from build123d import *

# Parameters (mm, degrees)
SKETCH_1_W          = 56
SKETCH_1_H          = 40
EXTRUDE_1_DEPTH     = 4
SKETCH_2_R          = 1.5
SKETCH_2_R_2        = 2.025
SKETCH_2_R_3        = 1.025
CUT_EXTRUDE_1_DEPTH = 34
EXTRUDE_2_DEPTH     = 4
SKETCH_4_R          = 1.525
CUT_EXTRUDE_2_DEPTH = 10
FILLET_1_R          = 2
CUT_EXTRUDE_3_DEPTH = 22
FILLET_2_R          = 2


with BuildPart() as part:
    # 草图1 → 凸台-拉伸1 (new body)
    with BuildSketch(Plane.XY):
        Rectangle(SKETCH_1_W, SKETCH_1_H)
    extrude(amount=EXTRUDE_1_DEPTH)

    # 草图2 → 切除-拉伸1 (cut)
    with BuildSketch(Plane(origin=(0, 0, 0), x_dir=(-1, 0, 0), z_dir=(0, 0, -1))):
        with Locations((3.7, 0)):
            Circle(SKETCH_2_R)
        with Locations((-25, 10)):
            Circle(SKETCH_2_R)
        with Locations((-25, -10)):
            Circle(SKETCH_2_R)
        with Locations((24.2, -12)):
            Circle(SKETCH_2_R_2)
        with Locations((24.2, 12)):
            Circle(SKETCH_2_R_2)
        with Locations((7.7, -9)):
            Circle(SKETCH_2_R_3)
        with Locations((15.7, -9)):
            Circle(SKETCH_2_R_3)
    extrude(amount=-CUT_EXTRUDE_1_DEPTH, mode=Mode.SUBTRACT)

    # 草图3 → 凸台-拉伸2 (add)
    with BuildSketch(Plane.XY.offset(4)):
        Polygon((28, 20), (-28, 70), (-28, 20), align=None)
    extrude_2 = extrude(amount=-EXTRUDE_2_DEPTH)

    # 镜向1: 凸台-拉伸2 across plane
    add(extrude_2.mirror(Plane.ZX))

    # 草图4 → 切除-拉伸2 (cut)
    with BuildSketch(Plane(origin=(0, 0, 0), x_dir=(-1, 0, 0), z_dir=(0, 0, -1))):
        with Locations((10.420660221, -47.601187919)):
            Circle(SKETCH_4_R)
        with Locations((-4.498093012, -34.280872533)):
            Circle(SKETCH_4_R)
    cut_extrude_2 = extrude(amount=-CUT_EXTRUDE_2_DEPTH, mode=Mode.SUBTRACT)

    # 镜向2: 切除-拉伸2 across plane
    add(cut_extrude_2.mirror(Plane.ZX), mode=Mode.SUBTRACT)

    # 圆角1
    fillet_1_edges = [part.edges().sort_by_distance(p)[0] for p in [
        (-28, 70, 2),
        (-28, -70, 2),
        (28, -20, 2),
        (28, 20, 2),
    ]]
    fillet(fillet_1_edges, radius=FILLET_1_R)

    # 草图5 → 切除-拉伸3 (cut)
    with BuildSketch(Plane(origin=(0, 0, 0), x_dir=(-1, 0, 0), z_dir=(0, 0, -1))):
        Polygon((-23, 7.185207752), (-2.378453751, 0), (-23, -7.185207752), align=None)
        Polygon((20.2, 52.310957498), (-24.014671549, 12.833572186), (4.207680626, 3), (20.2, 3), align=None)
        Polygon((4.207680626, -3), (20.2, -3), (20.2, -52.310957498), (-24.014671549, -12.833572186), align=None)
    extrude(amount=-CUT_EXTRUDE_3_DEPTH, mode=Mode.SUBTRACT)

    # 圆角2
    fillet_2_edges = [part.edges().sort_by_distance(p)[0] for p in [
        (24.014671549, -12.833572186, 2),
        (-4.207680626, -3, 2),
        (-20.2, -3, 2),
        (-20.2, -52.310957498, 2),
        (-20.2, 52.310957498, 2),
        (-20.2, 3, 2),
        (-4.207680626, 3, 2),
        (24.014671549, 12.833572186, 2),
        (23, -7.185207752, 2),
        (23, 7.185207752, 2),
        (2.378453751, 0, 2),
    ]]
    fillet(fillet_2_edges, radius=FILLET_2_R)


solid = part.part
Work out the finished part from the listing and answer in its coordinate system (mm). A direction names the side the tool comes from. Give positions to 0.01 mm unless a question says otherwise; leave off trailing zeros. Order: outer loops, then holes, each group sorted by start corner. A loop starts at its lowest first (then second) coordinate and runs counter-clockwise, first axis right, second up. Notation, with made-up numbers: (28, 29.25) -> (62, 29.25) arc R25 ccw to (62, 45.25) -> close; hole circle Ø11 at (17.25, -16). An arc over 180 degrees is marked (long way). Answer as a JSON object with one key per item and string values. Group by question number.
1. Consider line 1 along Y through (x, z) = (-25, 2.45); line 2 along Y through (x, z) = (4.5, 3); line 3 along Y through (x, z) = (10, 1.9). Determine where each line is inside the solid, lowest interval first. Write a range as [from, to].
2. Section C-C on y = 56.5 is taken. Determine the outline of the cut face in (x, z).
3. The mould has two halves that part along Y. Classify faces 1 (the cylindrical face through (-22.59, -13.23, 1.97)), 2 (the flat face through (-28, -1, 2)), 3 (the cylindrical face through (-26.847, 67.345, 1.972)), 4 (the cylindrical face through (6.457, -0.035, 2.028)): released by +Y, released by -Y, zero draft, split by the parting line, or undercut.
4. Section B-B on y = 25 is taken. Determine the outline of the cut face in (x, z).
5. Flat-ended cylindrical pins translate along their axes: pin 1 Ø1 at (y, z) = (-23.5, 1) entering from +X; pin 2 Ø1.2 at (x, z) = (-10, 2) entering from +Y; pin 3 Ø6.5 at (x, y) = (-24.2, 12) entering from +Z; pin 4 Ø1.2 at (x, z) = (-11, 1.5) entering from -Y. Find the tip coordinate at first contact, or state that the pin passes through.
6. A tool of negligible diameter and unlimited length cuts with its end or side. For faces 5 (the flat face through (-11, -3, 2)), 6 (the flat face through (-2, 0, 0)), from which of +Z, -Z, +X, -X, +Y, -Y can it reach the whole face along a straight path? Write none if from no direction.
7. Section D-D on z = 2.8 is taken. Count the separate pieces of the cut face and the enclosed holes in it, plus the area to 3 significant figures.
8. Section A-A on x = -0.5 is taken. Determine the outline of the cut face in (y, z), plus the area to 3 significant figures.
Result sheet:
{
 "1": {"line 1": "y = [-67.27, -13.86], [-10.14, 10.14], [13.86, 67.27]", "line 2": "y = [-40.98, -35.81], [-32.76, -30.26], [-6.03, 6.03], [30.26, 32.76], [35.81, 40.98]", "line 3": "y = [-36.07, -25.35], [-7.95, -2.66], [2.66, 7.95], [25.35, 36.07]"},
 "2": {"outline": "(-28, 0) -> (-12.88, 0) -> (-12.88, 4) -> (-28, 4) -> close"},
 "3": {"face 1": "undercut", "face 2": "zero draft", "face 3": "released by +Y", "face 4": "undercut"},
 "4": {"outline": "(-28, 0) -> (-20.2, 0) -> (-20.2, 4) -> (-28, 4) -> close; (10.39, 0) -> (22.4, 0) -> (22.4, 4) -> (10.39, 4) -> close"},
 "5": {"pin 1": "stops at x = 24.64", "pin 2": "stops at y = 54.46", "pin 3": "stops at z = 4", "pin 4": "stops at y = -55.36"},
 "6": {"face 5": "+Z, -Z", "face 6": "-Z, +X, -X, +Y, -Y"},
 "7": {"separate pieces": "1", "enclosed holes": "12", "area": "2,500 mm^2"},
 "8": {"outline": "(-45.45, 0) -> (-34.72, 0) -> (-34.72, 4) -> (-45.45, 4) -> close; (-4.29, 0) -> (4.29, 0) -> (4.29, 4) -> (-4.29, 4) -> close; (34.72, 0) -> (45.45, 0) -> (45.45, 4) -> (34.72, 4) -> close", "area": "120 mm^2"}
}
